```python
from build123d import *

# Parameters (mm, degrees)
SKETCH4_R           = 3
BOSS_EXTRUDE2_DEPTH = 10
SKETCH5_R           = 1.55
CUT_EXTRUDE1_DEPTH  = 11.4
BOSS_EXTRUDE3_START = 12
BOSS_EXTRUDE3_DEPTH = 12
CIRPATTERN2_COUNT   = 9


with BuildPart() as part:
    # Sketch1 → Revolve1 (revolve)
    with BuildSketch(Plane(origin=(0, 0, 0), x_dir=(1, 0, 0), z_dir=(0, 1, 0)), mode=Mode.PRIVATE) as revolve1_sk:
        with BuildLine():
            Line((0, 0), (0, 30))
            Line((0, 30), (-3, 30))
            Line((-3, 30), (-3, 5))
            Line((-3, 5), (-8, 5))
            ThreePointArc((-8, 5), (-10.828427125, 3.828427125), (-12, 1))
            Line((-12, 1), (-12, 0))
            Line((-12, 0), (0, 0))
        make_face()
    revolve(revolve1_sk.sketch.rotate(Axis((-12, 0, 0), (1, 0, 0)), 180), axis=Axis((-12, 0, 0), (1, 0, 0)))

    # Sketch4 → Boss-Extrude2 (add)
    with BuildSketch(Plane(origin=(0, 0, 0), x_dir=(0, 0, -1), z_dir=(1, 0, 0))):
        with Locations(Location((0, 0, 0), (0, 0, 180))):
            Circle(SKETCH4_R)
    extrude(amount=BOSS_EXTRUDE2_DEPTH)

    # Sketch5 → Cut-Extrude1 (cut)
    with BuildSketch(Plane(origin=(10, 0, 0), x_dir=(0, 0, -1), z_dir=(1, 0, 0))):
        Circle(SKETCH5_R)
    extrude(amount=-CUT_EXTRUDE1_DEPTH, mode=Mode.SUBTRACT)

    # Sketch6 → Boss-Extrude3 (add)
    with BuildSketch(Plane.ZY.offset(3).offset(BOSS_EXTRUDE3_START)):
        with BuildLine():
            ThreePointArc((8.265556015, 7.995660308), (7.604078802, 8.627165559), (6.89451328, 9.204112485))
            ThreePointArc((6.89451328, 9.204112485), (6.09737327, 21.594864355), (-3.195635958, 29.829312946))
            ThreePointArc((-3.195635958, 29.829312946), (-1.351457872, 29.969543901), (0.497856742, 29.995868693))
            ThreePointArc((0.497856742, 29.995868693), (8.428709352, 20.424655605), (8.265556015, 7.995660308))
        make_face()
    boss_extrude3 = extrude(amount=-BOSS_EXTRUDE3_DEPTH)

    # CirPattern2: Boss-Extrude3 ×9 about axis
    cirpattern2_axis = Axis((0, 0, 0), (1, 0, 0))
    for i in range(1, CIRPATTERN2_COUNT):
        add(boss_extrude3.rotate(cirpattern2_axis, i * 360 / CIRPATTERN2_COUNT))


solid = part.part
```
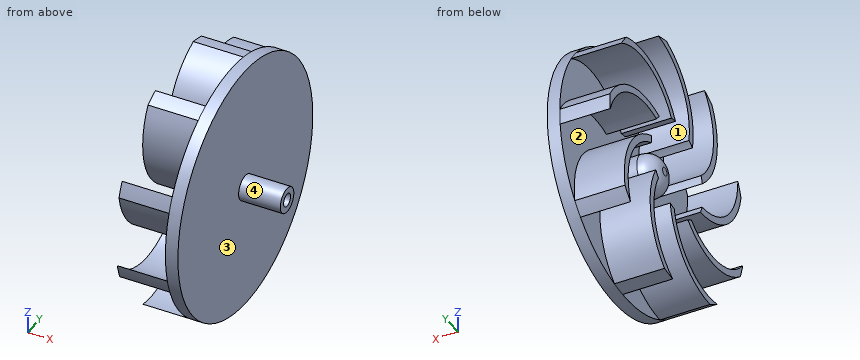
The listing builds one solid part. Answer for the finished solid, in the listing's coordinates (mm). Face numbers are marked on the shaded views. Coordinates: 2 decimals unless noted, no trailing zeros. Order: outer loops, then holes, each group sorted by start corner. A loop starts at its lowest first (then second) coordinate and runs counter-clockwise, first axis right, second up. Notation, with made-up numbers: M -22,-10.5 L -14,-10.5 A9 cw -14,6.5 Z; hole C 15.25,51 d1. An arc over 180 degrees is marked long. Answer as a JSON object with one key per item and string values. Group by question number.
1. Flat-ended cylindrical pins translate along their axes: P1, Ø2, axis at x = -4.5, y = -9, coming from the +Z side (3 decimals); P2, Ø0.9, axis at y = -0.5, z = 0.5, coming from the +X side; P3, Ø1, axis at x = -10, y = 14.5, coming from the +Z side. Find the tip coordinate at first contact, or state that the pin passes through.
2. Section C-C on y = 16.5 is taken. Write down the section's boundary in (x, z), then the cut area to 3 significant figures.
3. Determine the mould class of the marked faces 1, 2, 3 and 4 for opening direction Z: released by +Z, released by -Z, zero draft, split by the parting line, or undercut.
4. Section B-B on z = -17.5 is taken. Write down the section's boundary in (x, y).
5. Section D-D on x = -13 is taken. State how many separate pieces and enclosed holes the cut face has, then the cut area to 3 significant figures.
6. Section A-A on x = 8.25 is taken. Write down the section's boundary in (y, z).
7. Straight lines are drawn through the part: line 1 (Y direction, x = -10.5, z = -1); line 2 (Y direction, x = 4, z = 0); line 3 (Z direction, x = -10.75, y = 18.5). For each, find the intervals that lie inside material, in ascending order.
Values follow:
{
 "1": {"P1": "z = -10.825", "P2": "x = -1.4", "P3": "z = 20.66"},
 "2": {"outline": "M -15,-3.74 L -3,-3.74 L -3,-25.05 L 0,-25.05 L 0,25.05 L -3,25.05 L -3,20.73 L -15,20.73 L -15,19.03 L -3,19.03 L -3,9.34 L -15,9.34 L -15,7.62 L -3,7.62 L -3,-1.53 L -15,-1.53 Z", "area": "218 mm2"},
 "3": {"face 1": "undercut", "face 2": "undercut", "face 3": "zero draft", "face 4": "split by the parting line"},
 "4": {"outline": "M -15,-1.21 L -3,-1.21 L -3,-24.37 L 0,-24.37 L 0,24.37 L -3,24.37 L -3,23.48 L -15,23.48 L -15,21.78 L -3,21.78 L -3,12 L -15,12 L -15,10.29 L -3,10.29 L -3,0.81 L -15,0.81 Z"},
 "5": {"separate pieces": "9", "enclosed holes": "0", "area": "388 mm2"},
 "6": {"outline": "C 0,0 d6; hole C 0,0 d3.1"},
 "7": {"line 1": "-22 to -19.05, -4 to 4, 12.35 to 15.78, 28.88 to 29.98", "line 2": "-3 to -1.55, 1.55 to 3", "line 3": "-5.91 to -3.31, 7.24 to 8.99, 18.91 to 20.63"}
}
